from build123d import *

# Parameters (mm, degrees)
SKETCH1_R           = 1.75
EXTRUDE1_DEPTH      = 3.15
CHAMFER1_SIZE       = 1.5
EXTRUDE2_START      = 1.35
EXTRUDE2_DEPTH      = 1.35
EXTRUDE3_DEPTH      = 13.7
SKETCH4_W           = 5
SKETCH4_H           = 7
EXTRUDE4_DEPTH      = 3
SKETCH5_W           = 0.7
SKETCH5_H           = 4.8
EXTRUDE5_DEPTH      = 6.25
EXTRUDE6_DEPTH      = 17
FILLET1_R           = 0.5
SKETCH7_W           = 2
SKETCH7_H           = 4
EXTRUDE7_DEPTH      = 14
SKETCH8_W           = 2
SKETCH8_H           = 4
EXTRUDE8_DEPTH      = 16.5
CHAMFER3_SIZE       = 0.75
SKETCH9_W           = 0.7
SKETCH9_H           = 4.8
EXTRUDE9_DEPTH      = 7
FILLET2_R           = 2
EXTRUDE_THIN1_DEPTH = 2.5
EXTRUDE10_DEPTH     = 2
FILLET3_R           = 0.5
FILLET4_R           = 0.5
SKETCH13_W          = 24.5
SKETCH13_H          = 8.5
EXTRUDE11_DEPTH     = 0.5


with BuildPart() as part:
    # Sketch1 → Extrude1 (new body)
    with BuildSketch(Plane.XY):
        with BuildLine():
            Line((-12.75, 11.25), (12.75, 11.25))
            ThreePointArc((12.75, 11.25), (13.996574867, 10.917037402), (14.911099489, 10.00684088))
            Line((14.911099489, 10.00684088), (22.322198979, -2.73631824))
            ThreePointArc((22.322198979, -2.73631824), (23, -5.25), (22.322198979, -7.76368176))
            Line((22.322198979, -7.76368176), (14.911099489, -20.50684088))
            ThreePointArc((14.911099489, -20.50684088), (13.996574867, -21.417037402), (12.75, -21.75))
            Line((12.75, -21.75), (-12.75, -21.75))
            ThreePointArc((-12.75, -21.75), (-13.996574867, -21.417037402), (-14.911099489, -20.50684088))
            Line((-14.911099489, -20.50684088), (-22.322198979, -7.76368176))
            ThreePointArc((-22.322198979, -7.76368176), (-23, -5.25), (-22.322198979, -2.73631824))
            Line((-22.322198979, -2.73631824), (-14.911099489, 10.00684088))
            ThreePointArc((-14.911099489, 10.00684088), (-13.996574867, 10.917037402), (-12.75, 11.25))
        make_face()
        with Locations((-18, -5.25)):
            Circle(SKETCH1_R, mode=Mode.SUBTRACT)
        with Locations((18, -5.25)):
            Circle(SKETCH1_R, mode=Mode.SUBTRACT)
    extrude(amount=EXTRUDE1_DEPTH)

    # Chamfer1
    chamfer1_edges = [part.edges().sort_by_distance(p)[0] for p in [
        (-19.75, -5.25, 0),
        (16.25, -5.25, 0),
    ]]
    chamfer(chamfer1_edges, length=CHAMFER1_SIZE)

    # Sketch2 → Extrude2 (add)
    with BuildSketch(Plane(origin=(0, 0, 0), x_dir=(-1, 0, 0), z_dir=(0, 0, -1)).offset(EXTRUDE2_START)):
        with BuildLine():
            Line((-12.75, 11.25), (12.75, 11.25))
            ThreePointArc((12.75, 11.25), (14.517766953, 10.517766953), (15.25, 8.75))
            Line((15.25, 8.75), (15.25, -19.25))
            ThreePointArc((15.25, -19.25), (14.517766953, -21.017766953), (12.75, -21.75))
            Line((12.75, -21.75), (-12.75, -21.75))
            ThreePointArc((-12.75, -21.75), (-14.517766953, -21.017766953), (-15.25, -19.25))
            Line((-15.25, -19.25), (-15.25, 8.75))
            ThreePointArc((-15.25, 8.75), (-14.517766953, 10.517766953), (-12.75, 11.25))
        make_face()
    extrude(amount=-EXTRUDE2_DEPTH)

    # Sketch3 → Extrude3 (add)
    with BuildSketch(Plane.XY.offset(3.15)):
        with BuildLine():
            Line((-7.75, 9.5), (7.75, 9.5))
            Line((7.75, 9.5), (13.25, 4))
            Line((13.25, 4), (13.25, -16.5))
            ThreePointArc((13.25, -16.5), (12.078427125, -19.328427125), (9.25, -20.5))
            Line((9.25, -20.5), (-9.25, -20.5))
            ThreePointArc((-9.25, -20.5), (-12.078427125, -19.328427125), (-13.25, -16.5))
            Line((-13.25, -16.5), (-13.25, 4))
            Line((-13.25, 4), (-7.75, 9.5))
        make_face()
    extrude(amount=EXTRUDE3_DEPTH)

    # Sketch4 → Extrude4 (add)
    with BuildSketch(Plane.XY.offset(16.85)):
        with Locations((-7, -3.5)):
            Rectangle(SKETCH4_W, SKETCH4_H)
        with Locations((0, 3.5)):
            Rectangle(SKETCH4_W, SKETCH4_H)
        with Locations((7, -3.5)):
            Rectangle(SKETCH4_W, SKETCH4_H)
    extrude(amount=EXTRUDE4_DEPTH)

    # Sketch5 → Extrude5 (add)
    with BuildSketch(Plane.XY.offset(19.85)):
        with Locations((0, 3.5)):
            Rectangle(SKETCH5_W, SKETCH5_H)
        with Locations((7, -3.5)):
            Rectangle(SKETCH5_W, SKETCH5_H)
        with Locations((-7, -3.5)):
            Rectangle(SKETCH5_W, SKETCH5_H)
    extrude(amount=EXTRUDE5_DEPTH)

    # Sketch6 → Extrude6 (cut)
    with BuildSketch(Plane(origin=(0, 0, -1.35), x_dir=(-1, 0, 0), z_dir=(0, 0, -1))):
        with BuildLine():
            Line((-6.7, 7.85), (6.7, 7.85))
            Line((6.7, 7.85), (12.2, 2.35))
            Line((12.2, 2.35), (12.2, -5.35))
            ThreePointArc((12.2, -5.35), (11.467766953, -7.117766953), (9.7, -7.85))
            Line((9.7, -7.85), (-9.7, -7.85))
            ThreePointArc((-9.7, -7.85), (-11.467766953, -7.117766953), (-12.2, -5.35))
            Line((-12.2, -5.35), (-12.2, 2.35))
            Line((-12.2, 2.35), (-6.7, 7.85))
        make_face()
    extrude(amount=-EXTRUDE6_DEPTH, mode=Mode.SUBTRACT)

    # Fillet1
    fillet1_edges = [part.edges().sort_by_distance(p)[0] for p in [
        (9.45, 5.1, -1.35),
        (12.2, -1.5, -1.35),
        (11.467766953, -7.117766953, -1.35),
        (0, -7.85, -1.35),
        (-11.467766953, -7.117766953, -1.35),
        (-12.2, -1.5, -1.35),
        (-9.45, 5.1, -1.35),
        (0, 7.85, -1.35),
    ]]
    fillet(fillet1_edges, radius=FILLET1_R)

    # Sketch7 → Extrude7 (add)
    with BuildSketch(Plane(origin=(0, 0, 15.65), x_dir=(-1, 0, 0), z_dir=(0, 0, -1))):
        with Locations((-7, -2)):
            Rectangle(SKETCH7_W, SKETCH7_H)
        with Locations((7, -2)):
            Rectangle(SKETCH7_W, SKETCH7_H)
    extrude(amount=EXTRUDE7_DEPTH)

    # Sketch8 → Extrude8 (add)
    with BuildSketch(Plane(origin=(0, 0, 15.65), x_dir=(-1, 0, 0), z_dir=(0, 0, -1))):
        with Locations((0, 2)):
            Rectangle(SKETCH8_W, SKETCH8_H)
    extrude(amount=EXTRUDE8_DEPTH)

    # Chamfer3
    chamfer3_edges = [part.edges().sort_by_distance(p)[0] for p in [
        (8, -2, 1.65),
        (7, -4, 1.65),
        (6, -2, 1.65),
        (7, 0, 1.65),
        (-6, -2, 1.65),
        (-7, -4, 1.65),
        (-8, -2, 1.65),
        (-7, 0, 1.65),
        (1, 2, -0.85),
        (0, 0, -0.85),
        (-1, 2, -0.85),
        (0, 4, -0.85),
    ]]
    chamfer(chamfer3_edges, length=CHAMFER3_SIZE)

    # Sketch9 → Extrude9 (add)
    with BuildSketch(Plane.XY.offset(16.85)):
        with Locations((-5.85, -13.4)):
            Rectangle(SKETCH9_W, SKETCH9_H)
        with Locations((5.85, -13.4)):
            Rectangle(SKETCH9_W, SKETCH9_H)
    extrude(amount=EXTRUDE9_DEPTH)

    # Fillet2
    fillet2_edges = [part.edges().sort_by_distance(p)[0] for p in [
        (0, 1.1, 26.1),
        (0, 5.9, 26.1),
        (7, -5.9, 26.1),
        (7, -1.1, 26.1),
        (-7, -5.9, 26.1),
        (-7, -1.1, 26.1),
        (-5.85, -15.8, 23.85),
        (-5.85, -11, 23.85),
        (5.85, -15.8, 23.85),
        (5.85, -11, 23.85),
    ]]
    fillet(fillet2_edges, radius=FILLET2_R)

    # Sketch10 → Extrude-Thin1 (add, symmetric)
    with BuildSketch(Plane(origin=(6, 0, 0), x_dir=(0, 0, -1), z_dir=(1, 0, 0))):
        with BuildLine():
            Line((-20, 0), (-20, -7.5))
            ThreePointArc((-20, -7.5), (-19.766044443, -8.14278761), (-19.173648178, -8.484807753))
            Line((-19.173648178, -8.484807753), (-18.826351822, -8.546045471))
            ThreePointArc((-18.826351822, -8.546045471), (-18.233955557, -8.888065614), (-18, -9.530853224))
            Line((-18, -9.530853224), (-18, -17))
            Line((-18, -17), (-18.5, -17))
            Line((-18.5, -17), (-18.5, -9.530853224))
            ThreePointArc((-18.5, -9.530853224), (-18.616977778, -9.209459419), (-18.913175911, -9.038449347))
            Line((-18.913175911, -9.038449347), (-19.260472267, -8.97721163))
            ThreePointArc((-19.260472267, -8.97721163), (-20.149066665, -8.464181415), (-20.5, -7.5))
            Line((-20.5, -7.5), (-20.5, 0))
            Line((-20.5, 0), (-20, 0))
        make_face()
    extrude(amount=EXTRUDE_THIN1_DEPTH, both=True)

    # Sketch12 → Extrude10 (cut)
    with BuildSketch(Plane(origin=(7.35, 0, 0), x_dir=(0, 0, -1), z_dir=(1, 0, 0))):
        Polygon((-21, -1.1), (-21, -10.028067218), (-19, -10.028067218), (-19, -16.1), (-27, -16.1), (-27, -1.1), align=None)
    extrude(amount=-EXTRUDE10_DEPTH, mode=Mode.SUBTRACT)

    # Fillet3
    fillet3_edges = [part.edges().sort_by_distance(p)[0] for p in [
        (5.85, -11, 18.5),
        (5.5, -13.4, 18.5),
        (5.85, -15.8, 18.5),
        (6.2, -13.4, 18.5),
    ]]
    fillet(fillet3_edges, radius=FILLET3_R - 0.0001)  # a hair under: the kernel refuses the full size

    # Fillet4
    fillet4_edges = [part.edges().sort_by_distance(p)[0] for p in [
        (7, -1.1, 20.5),
        (6.65, -3.5, 20.5),
        (7, -5.9, 20.5),
        (7.35, -3.5, 20.5),
    ]]
    fillet(fillet4_edges, radius=FILLET4_R - 0.0001)  # a hair under: the kernel refuses the full size

    # Sketch13 → Extrude11 (add)
    with BuildSketch(Plane(origin=(0, 0, -1.35), x_dir=(-1, 0, 0), z_dir=(0, 0, -1))):
        with Locations((0, -14.25)):
            Rectangle(SKETCH13_W, SKETCH13_H)
    extrude(amount=EXTRUDE11_DEPTH)


solid = part.part
Could you check a few things on this model? Use its own coordinates, in mm. A direction names the side the tool comes from. Give positions to 0.01 mm unless a question says otherwise; leave off trailing zeros. Order: outer loops, then holes, each group sorted by start corner. A loop starts at its lowest first (then second) coordinate and runs counter-clockwise, first axis right, second up. Notation, with made-up numbers: (68, 56.25) - (121, 56.25) arc R34 cw to (121, 86.25) - close; hole circle Ø7 at (5.25, -23.75). An arc over 180 degrees is marked (long way). One line per item, written item: value. Start each with the question number.
1. Imagine slicing it at B-B on z = 0.75. List the corners of the cut face in (x, y) for me, plus the area to 3 significant figures.
2. For P1, Ø1.5, axis at x = -6.5, z = 6.5, coming from the +Y side; P2, Ø1.5, axis at x = -6.5, z = 18.5, coming from the +Y side; P3, Ø1.5, axis at y = 2, z = 19, coming from the -X side, each with a flat end and sliding along its axis, tell me the tip position at first contact or that it passes through.
3. If I drill on probe 1 along X at (y, z) = (1.5, 7.5); probe 2 along X at (y, z) = (-5, 1.75); probe 3 along Y at (x, z) = (4, 12.5), over which ranges is the centre line in solid material (lowest first)?
4. Thinking about a two-plate mould opening in X: for faces 5 (the face through (0, 5.33, 25.5)), 6 (the face through (-23, -5.3, 1.6)), 7 (the face through (-9.6, 5.17, -1.21)), 8 (the face through (6.2, -13.4, 17.4)), which applies, +X half, -X half, draft (parallel to the pull), parting line (faces both ways), or undercut?
5. Imagine slicing it at A-A on z = 5.25. List the corners of the cut face in (x, y) for me.
6. Imagine slicing it at C-C on x = 18. List the corners of the cut face in (y, z) for me, plus the area to 3 significant figures.
7. For faces 1 (the face through (-5.5, -13, 20)), 2 (the face through (8, -2, 9)), 3 (the face through (-7.35, -4, 23)), 4 (the face through (10.46, 6.79, 9.9)), which set-ups out of +Z, -Z, +X, -X, +Y, -Y let a thin tool reach every point of the face, with its end or its side?
Values:
1. outline: (-22.32, -7.76) - (-14.91, -20.51) arc R2.5 ccw to (-12.75, -21.75) - (12.75, -21.75) arc R2.5 ccw to (14.91, -20.51) - (22.32, -7.76) arc R5 ccw to (22.32, -2.74) - (14.91, 10.01) arc R2.5 ccw to (12.75, 11.25) - (-12.75, 11.25) arc R2.5 ccw to (-14.91, 10.01) - (-22.32, -2.74) arc R5 ccw to start; (-1, 0) - (1, 0) - (1, 4) - (-1, 4) - close; hole circle Ø5 at (-18, -5.25); hole (-12.2, -5.35) arc R2.5 ccw to (-9.7, -7.85) - (9.7, -7.85) arc R2.5 ccw to (12.2, -5.35) - (12.2, 2.35) - (6.7, 7.85) - (-6.7, 7.85) - (-12.2, 2.35) - close; hole circle Ø5 at (18, -5.25)
1. area: 868 mm²
2. P1: y = 9.5
2. P2: y = 0
2. P3: x = -2.5
3. probe 1: -13.25 to -12.2, -1 to 1, 12.2 to 13.25
3. probe 2: -22.99 to -19.73, -16.27 to -12.2, 12.2 to 16.27, 19.73 to 22.99
3. probe 3: -20.5 to -7.85, 7.85 to 9.5
4. face 5: draft
4. face 6: -X half
4. face 7: undercut
4. face 8: +X half
5. outline: (-13.25, -16.5) arc R4 ccw to (-9.25, -20.5) - (9.25, -20.5) arc R4 ccw to (13.25, -16.5) - (13.25, 4) - (7.75, 9.5) - (-7.75, 9.5) - (-13.25, 4) - close; (-8, -4) - (-6, -4) - (-6, 0) - (-8, 0) - close; (-1, 0) - (1, 0) - (1, 4) - (-1, 4) - close; (6, -4) - (8, -4) - (8, 0) - (6, 0) - close; hole (-12.2, -5.35) arc R2.5 ccw to (-9.7, -7.85) - (9.7, -7.85) arc R2.5 ccw to (12.2, -5.35) - (12.2, 2.35) - (6.7, 7.85) - (-6.7, 7.85) - (-12.2, 2.35) - close
6. outline: (-15.2, 0) - (-8.5, 0) - (-7, 1.5) - (-7, 3.15) - (-15.2, 3.15) - close; (-3.5, 1.5) - (-2, 0) - (4.7, 0) - (4.7, 3.15) - (-3.5, 3.15) - close
6. area: 49.4 mm²
7. face 1: +Z, -Y
7. face 2: -Z
7. face 3: +Z, -X, +Y, -Y
7. face 4: +Z, +X, +Y
